Geometry: final body of the model. Coordinates: model frame, mm. A direction names the side the tool comes from. Give positions to 0.01 mm unless a question says otherwise; leave off trailing zeros. Write each loop counter-clockwise with the first axis right and the second up, starting at its lowest first coordinate (ties: lowest second). Pieces come first, ordered by that corner, then holes.
```python
from build123d import *

# Parameters (mm, degrees)
SKETCH2_W                = 70
SKETCH2_H                = 55
BOSS_EXTRUDE3_DEPTH      = 3
BOSS_EXTRUDE4_DEPTH      = 10
BOSS_EXTRUDE4_DEPTH_BACK = 10
SKETCH5_W                = 5
SKETCH5_H                = 55
SKETCH6_W                = 40
SKETCH6_H                = 55
BOSS_EXTRUDE5_DEPTH      = 3
SKETCH8_W                = 3
SKETCH8_H                = 8
BOSS_EXTRUDE6_DEPTH      = 11
SKETCH9_R                = 1.6
CUT_EXTRUDE1_DEPTH       = 11


with BuildPart() as part:
    # Sketch2 → Boss-Extrude3 (new body)
    with BuildSketch(Plane(origin=(0, 0, 0), x_dir=(1, 0, 0), z_dir=(0, 1, 0))):
        with Locations((4.454545455, 9.045454545)):
            Rectangle(SKETCH2_W, SKETCH2_H)
    extrude(amount=BOSS_EXTRUDE3_DEPTH)

    # Sketch5 → Boss-Extrude4 (add, two sides: drawn at the far end of the back side and taken through both)
    with BuildSketch(Plane(origin=(0, 0, 0), x_dir=(1, 0, 0), z_dir=(0, 1, 0)).offset(-BOSS_EXTRUDE4_DEPTH_BACK)):
        with Locations((41.954545455, 9.045454545)):
            Rectangle(SKETCH5_W, SKETCH5_H)
    extrude(amount=BOSS_EXTRUDE4_DEPTH + BOSS_EXTRUDE4_DEPTH_BACK)

    # Sketch6 → Boss-Extrude5 (add)
    with BuildSketch(Plane(origin=(0, 0, 0), x_dir=(1, 0, 0), z_dir=(0, 1, 0))):
        with Locations((64.454545455, 9.045454545)):
            Rectangle(SKETCH6_W, SKETCH6_H)
    extrude(amount=BOSS_EXTRUDE5_DEPTH)

    # Sketch8 → Boss-Extrude6 (add)
    with BuildSketch(Plane(origin=(0, 0, 0), x_dir=(1, 0, 0), z_dir=(0, 1, 0))):
        with Locations((82.954545455, 22.045454545)):
            Rectangle(SKETCH8_W, SKETCH8_H)
        with Locations((82.954545455, -3.954545455)):
            Rectangle(SKETCH8_W, SKETCH8_H)
    extrude(amount=BOSS_EXTRUDE6_DEPTH)

    # Sketch9 → Cut-Extrude1 (cut)
    with BuildSketch(Plane(origin=(84.454545455, 0, 0), x_dir=(0, 0, -1), z_dir=(1, 0, 0))):
        with Locations((-2.704545455, 8.25)):
            Circle(SKETCH9_R)
        with Locations((20.795454545, 8.25)):
            Circle(SKETCH9_R)
    extrude(amount=-CUT_EXTRUDE1_DEPTH, mode=Mode.SUBTRACT)


solid = part.part
```
Item 1: Line query: L1, parallel to X at y = 5.75, z = -21; L2, parallel to Y at x = -10.5, z = -26; L3, parallel to X at y = 7.25, z = -7. Output: solid intervals per line, ascending.
Found:
L1: x = 39.45 to 44.45, 81.45 to 84.45
L2: y = 0 to 3
L3: x = 39.45 to 44.45
Item 2: Reachability of faces 4 (the face through (83, 6.7, 3.1)), 5 (the face through (4, 3, -9)), 6 (the face through (64, 0, -9)) from +Z, -Z, +X, -X, +Y, -Y: full face, straight path, thin tool, end or side. Return the list, or none.
Found:
face 4: +X
face 5: +Z, -Z, -X, +Y
face 6: +Z, -Z, +X, -Y
Item 3: Pin query (flat end, axial travel): pin 1 Ø1.9 at (y, z) = (8.25, -20.8) entering from -X; pin 2 Ø1.5 at (x, z) = (53.5, -16.5) entering from +Y; pin 3 Ø2.5 at (x, y) = (83.5, 6.5) entering from +Z. Return the tip coordinate at first contact, or that it passes through.
Found:
pin 1: stops at x = 39.45
pin 2: stops at y = 3
pin 3: stops at z = 7.95
Item 4: Section B-B, the plane z = -6. Return the cut outline in (x, y), plus the area to 3 significant figures.
Found:
outline: (-30.55, 0) - (39.45, 0) - (39.45, -10) - (44.45, -10) - (44.45, 0) - (84.45, 0) - (84.45, 3) - (44.45, 3) - (44.45, 10) - (39.45, 10) - (39.45, 3) - (-30.55, 3) - close
area: 430 mm2
Item 5: Section C-C, the plane z = 3. Return the cut outline in (x, y), plus the area to 3 significant figures.
Found:
outline: (-30.55, 0) - (39.45, 0) - (39.45, -10) - (44.45, -10) - (44.45, 0) - (84.45, 0) - (84.45, 6.68) - (81.45, 6.68) - (81.45, 3) - (44.45, 3) - (44.45, 10) - (39.45, 10) - (39.45, 3) - (-30.55, 3) - close; (81.45, 9.82) - (84.45, 9.82) - (84.45, 11) - (81.45, 11) - close
area: 445 mm2
Item 6: Pull-direction query (Z, two-part tool) for faces 1 (the face through (44.455, 6, -9)), 2 (the face through (83, 7, -18.045)), 3 (the face through (31, 1, 18.455)); classes: +Z half, -Z half, draft (parallel to the pull), parting line (faces both ways), or undercut.
Found:
face 1: draft
face 2: undercut
face 3: +Z half
Item 7: Section D-D, the plane x = 13. Return the cut outline in (y, z).
Found:
outline: (0, -36.55) - (3, -36.55) - (3, 18.45) - (0, 18.45) - close
Item 8: Section A-A, the plane y = 8.25. Return the cut outline in (x, z), plus the area to 3 significant figures.
Found:
outline: (39.45, -36.55) - (44.45, -36.55) - (44.45, 18.45) - (39.45, 18.45) - close; (81.45, -26.05) - (84.45, -26.05) - (84.45, -22.4) - (81.45, -22.4) - close; (81.45, -19.2) - (84.45, -19.2) - (84.45, -18.05) - (81.45, -18.05) - close; (81.45, -0.05) - (84.45, -0.05) - (84.45, 1.1) - (81.45, 1.1) - close; (81.45, 4.3) - (84.45, 4.3) - (84.45, 7.95) - (81.45, 7.95) - close
area: 304 mm2
